Build history of the part. All positions in model axes, mm. Face numbers are marked on the shaded views. A direction names the side the tool comes from. Round coordinates to 2 decimals unless told otherwise and drop trailing zeros. Loops run counter-clockwise (first coordinate to the right, second up) from the corner with the lowest first, then second, coordinate; pieces in that order, holes last. Notation, with made-up numbers: (30.5, 39) -> (66.5, 39) arc R38 ccw to (66.5, 77) -> close; hole circle Ø11 at (-8.5, 42.25). An arc over 180 degrees is marked (long way). Put each result on its own line as item: value. Start each with the question number.
Item 1: Cut at A-A, the plane z = 6. List the corners of the cut face in (x, y).
Item 2: Tool access for the marked faces 1, 2 and 3: list every direction of +Z, -Z, +X, -X, +Y, -Y with a clear straight run to the whole face (end or side of a thin tool).
Item 3: Flat gauge pins, fed straight in: pin 1 Ø4.5 at (x, z) = (-42.5, 1) entering from -Y; pin 2 Ø1.5 at (y, z) = (-11, -5) entering from +X; pin 3 Ø4.5 at (y, z) = (-9, 1) entering from -X. Where does each tip first touch, or does it go through?
Item 4: Cut at B-B, the plane y = -13.5. List the corners of the cut face in (x, z), plus the area to 3 significant figures.
Item 5: Drill centre lines: probe 1 along Y at (x, z) = (29, 4.25); probe 2 along X at (y, z) = (-21.5, -3.75). Where is each one in solid material? Low to high. Write a range as [from, to].
Item 6: Cut at C-C, the plane x = 31. List the corners of the cut face in (y, z).
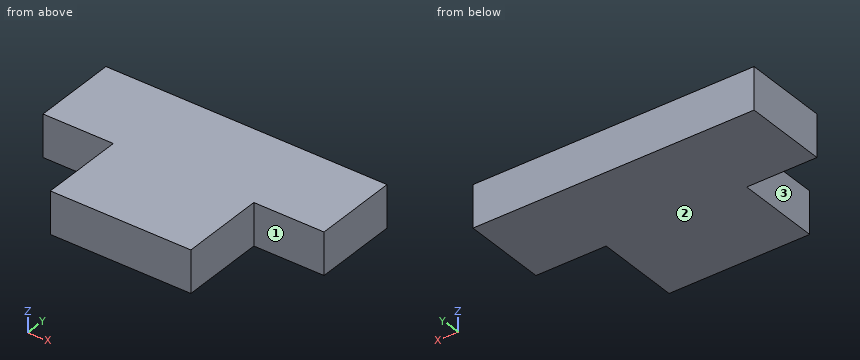
```python
from build123d import *

# Parameters (mm, degrees)
PLAT_W                      = 60
PLAT_H                      = 15
EL_MENT_M_CANO_SOUD_1_DEPTH = 100
ESQUISSE2_W                 = 25
ESQUISSE2_H                 = 30
ENL_V_MAT_EXTRU_1_DEPTH     = 20


with BuildPart() as part:
    # plat → Elément mécano-soudé1 (new body)
    with BuildSketch(Plane.YZ.offset(-50)):
        Rectangle(PLAT_W, PLAT_H)
    extrude(amount=EL_MENT_M_CANO_SOUD_1_DEPTH)

    # Esquisse2 → Enlèv. mat.-Extru.1 (cut)
    with BuildSketch(Plane.XY.offset(7.5)):
        with Locations((-37.5, -15)):
            Rectangle(ESQUISSE2_W, ESQUISSE2_H)
        with Locations((37.5, -15)):
            Rectangle(ESQUISSE2_W, ESQUISSE2_H)
    extrude(amount=-ENL_V_MAT_EXTRU_1_DEPTH, mode=Mode.SUBTRACT)


solid = part.part
```
Reply:
1. outline: (-50, 0) -> (-25, 0) -> (-25, -30) -> (25, -30) -> (25, 0) -> (50, 0) -> (50, 30) -> (-50, 30) -> close
2. face 1: +Z, -Z, +X, -Y
2. face 2: -Z, +X, -X, +Y, -Y
2. face 3: +Z, -Z, -X, -Y
3. pin 1: stops at y = 0
3. pin 2: stops at x = 25
3. pin 3: stops at x = -25
4. outline: (-25, -7.5) -> (25, -7.5) -> (25, 7.5) -> (-25, 7.5) -> close
4. area: 750 mm^2
5. probe 1: y = [0, 30]
5. probe 2: x = [-25, 25]
6. outline: (0, -7.5) -> (30, -7.5) -> (30, 7.5) -> (0, 7.5) -> close
